from build123d import *

# Parameters (mm, degrees)
F0_W          = 69.85
F0_H          = 6.35
F2_W          = 50.8
F2_H          = 6.35
F5_DEPTH      = 6.35
F7_DEPTH      = 6.35
F9_DEPTH      = 3.8354
F10_T4_DEPTH  = 70.8999806704
F10_T10_DEPTH = 72.2676909626
F11_W         = 69.85
F11_H         = 6.35
F12_DEPTH     = 6.35
F13_W         = 50.8
F13_H         = 6.35
F14_DEPTH     = 50.8
F15_SIZE      = 6.34999
F16_W         = 19.05
F16_H         = 19.05
F17_DEPTH     = 57.15
F18_W         = 19.05
F18_H         = 19.05
F19_DEPTH     = 111.76
F20_SIZE      = 6.34999
F21_R         = 3.175
F22_DEPTH     = 25.4


# Not quite as in the source:
# - a fillet or chamfer that OpenCascade refuses, or shapes differently, is made with other operations: its cross-section is extruded or revolved along the edge and cut away or added
# - a fillet or chamfer is up to 0.001 mm smaller than in the source, because OpenCascade refuses the exact size


with BuildPart() as f3:
    # F0 (on Front) → F3 section 0
    with BuildSketch(Plane.XZ):
        with Locations((-34.925, 3.175)):
            Rectangle(F0_W, F0_H)
    # F2 (on offset) → F3 section 1
    with BuildSketch(Plane.XZ.offset(82.55)):
        with Locations((-34.925, -28.575)):
            Rectangle(F2_W, F2_H)
    loft()

    # F4 (on face) → F5 (join)
    with BuildSketch(Plane(origin=(-68.9322627737, -7.9537226277, 0), x_dir=(0.114624108, -0.9934089359, 0), z_dir=(-0.9934089359, -0.114624108, 0))):
        Polygon((-8.0064939428, 31.75), (-8.0064939428, 6.35), (-8.0064939428, 0), (75.091208342, -31.75), (75.091208342, -25.4), (75.091208342, 0), align=None)
    extrude(amount=F5_DEPTH)

    # F6 (on face) → F7 (join)
    with BuildSketch(Plane(origin=(0, 0, 0), x_dir=(0.114624108, 0.9934089359, 0), z_dir=(0.9934089359, -0.114624108, 0))):
        Polygon((-83.0977022847, 0), (-83.0977022847, -31.75), (0, 0), (0, 31.75), align=None)
    extrude(amount=F7_DEPTH)

    # F8 (on face) → F9 (join)
    with BuildSketch(Plane(origin=(0, -2.1275773196, 5.5317010309), x_dir=(1, 0, 0), z_dir=(0, -0.3589790793, 0.9333456062))):
        Polygon((-61.6927102922, -73.4657484065), (-61.0088551461, -79.8157484065), (-8.8411448539, -79.8157484065), (-8.1572897078, -73.4657484065), align=None)
    extrude(amount=F9_DEPTH)

    # F10: fillet of radius 3.81 on 2 edges, made by hand


with BuildPart() as f10_tool2:
    # F10_s3 → F10_t4 (new body)
    with BuildSketch(Plane.YZ.offset(-70.3749903352)):
        with BuildLine():
            ThreePointArc((-76.6323734692, -23.096775868), (-76.5579487098, -20.1816780202), (-74.4440370018, -18.1730188162))
            Line((-74.4440370018, -18.1730188162), (-78.0000837614, -19.5407291084))
            Line((-78.0000837614, -19.5407291084), (-76.6323734692, -23.096775868))
        make_face()
    extrude(amount=F10_T4_DEPTH)

    split(bisect_by=Plane(origin=(0, 0, 0), x_dir=(0, 0, 1), z_dir=(-0.9934089359, 0.114624108, 0)), keep=Keep.TOP)

    split(bisect_by=Plane(origin=(-68.9322627737, -7.9537226277, 0), x_dir=(0, 0, 1), z_dir=(0.9934089359, 0.114624108, 0)), keep=Keep.TOP)


with BuildPart() as f3_1:
    add(f3.part)

    # F10_t1: cut F10_tool2
    add(f10_tool2.part, mode=Mode.SUBTRACT)


with BuildPart() as f10_tool8:
    # F10_s9 → F10_t10 (new body)
    with BuildSketch(Plane.YZ.offset(1.2088454813)):
        with BuildLine():
            ThreePointArc((-70.7056288698, -20.8172587144), (-72.7142880738, -18.7033470063), (-75.6293859216, -18.6289222469))
            Line((-75.6293859216, -18.6289222469), (-72.073339162, -17.2612119547))
            Line((-72.073339162, -17.2612119547), (-70.7056288698, -20.8172587144))
        make_face()
    extrude(amount=-F10_T10_DEPTH)

    split(bisect_by=Plane(origin=(0, 0, 0), x_dir=(0, 0, 1), z_dir=(-0.9934089359, 0.114624108, 0)), keep=Keep.TOP)

    split(bisect_by=Plane(origin=(-68.9322627737, -7.9537226277, 0), x_dir=(0, 0, 1), z_dir=(0.9934089359, 0.114624108, 0)), keep=Keep.TOP)


with BuildPart() as f3_2:
    add(f3_1.part)

    # F10_t7: cut F10_tool8
    add(f10_tool8.part, mode=Mode.SUBTRACT)

    # F11 (on face) → F12 (join)
    with BuildSketch(Plane(origin=(0, 0, 0), x_dir=(-1, 0, 0), z_dir=(0, 1, 0))):
        with Locations((34.925, 3.175)):
            Rectangle(F11_W, F11_H)
    extrude(amount=F12_DEPTH)

    # F13 (on face) → F14 (join)
    with BuildSketch(Plane.XY.offset(6.35)):
        with Locations((-34.925, 3.175)):
            Rectangle(F13_W, F13_H)
    extrude(amount=F14_DEPTH)

    # F15 (size 6.35 in the source; OpenCascade refuses exactly that, so slightly less here)
    f15_edges = [f3_2.edges().sort_by_distance(p)[0] for p in [
        (-34.925, 0, 57.15),
    ]]
    chamfer(f15_edges, length=F15_SIZE)

    # F16 (on face) → F17 (join)
    with BuildSketch(Plane(origin=(0, 6.35, 0), x_dir=(-1, 0, 0), z_dir=(0, 1, 0))):
        with Locations((34.925, 15.875)):
            Rectangle(F16_W, F16_H)
    extrude(amount=F17_DEPTH)

    # F18 (on face) → F19 (join)
    with BuildSketch(Plane.YZ.offset(-25.4)):
        with Locations((53.975, 15.875)):
            Rectangle(F18_W, F18_H)
    extrude(amount=F19_DEPTH)

    # F20 (size 6.35 in the source; OpenCascade refuses exactly that, so slightly less here)
    f20_edges = [f3_2.edges().sort_by_distance(p)[0] for p in [
        (-65.0875, -41.275, 15.875),
        (-4.7625, -41.275, 15.875),
    ]]
    chamfer(f20_edges, length=F20_SIZE)

    # F21 (on face) → F22 (cut)
    with BuildSketch(Plane.YZ.offset(86.36)):
        with Locations((53.975, 15.875)):
            Circle(F21_R)
    extrude(amount=-F22_DEPTH, mode=Mode.SUBTRACT)


solid = f3_2.part
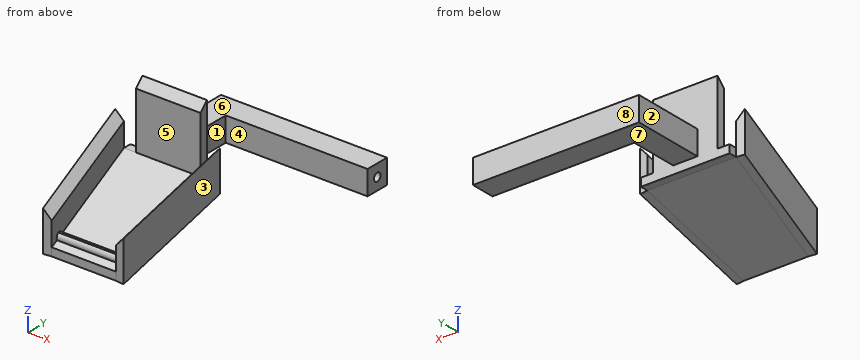
Geometry check sheet. Reference: the model listing, model coordinates, mm. Face numbers are marked on the shaded views. A direction names the side the tool comes from. Round coordinates to 2 decimals unless told otherwise and drop trailing zeros. Write each loop counter-clockwise with the first axis right and the second up, starting at its lowest first coordinate (ties: lowest second). Pieces come first, ordered by that corner, then holes.
Item 1: Section check B-B (x = 23). Record the boundary of the cut face in (y, z).
Determined:
outline: (44.45, 6.35) - (63.5, 6.35) - (63.5, 25.4) - (44.45, 25.4) - close
Item 2: Section check A-A (z = 21.5). Give the number of separate pieces and of enclosed holes in the cut face, plus the area to 3 significant figures.
Determined:
separate pieces: 3
enclosed holes: 0
area: 3,770 mm2
Item 3: Go/stop test with flat-tipped pins: pin 1 Ø7 at (x, y) = (-4.5, 3) entering from +Z; pin 2 Ø8 at (x, y) = (-41, -2.5) entering from +Z; pin 3 Ø5.5 at (y, z) = (21.5, 14) entering from -X. Record where each tip stops, or that it passes through.
Determined:
pin 1: stops at z = 6.35
pin 2: stops at z = 52.3
pin 3: stops at x = -44.45
Item 4: Section check C-C (y = 42.5). Record the boundary of the cut face in (x, z).
Determined:
outline: (-44.45, 6.35) - (-25.4, 6.35) - (-25.4, 25.4) - (-44.45, 25.4) - close
Item 5: Mould release check, pull along Y, two halves, no side actions. Record for the marked faces 1, 2, 3 and 4: +Y half, -Y half, draft (parallel to the pull), parting line (faces both ways), or undercut.
Determined:
face 1: undercut
face 2: draft
face 3: -Y half
face 4: undercut
Item 6: Material ranges on line 1 along X through (y, z) = (48, 10.5); line 2 along Z through (x, y) = (30.5, 51.5); line 3 along X through (y, z) = (-48.5, 0.5), recorded low to high.
Determined:
line 1: x = -44.45 to 86.36
line 2: z = 6.35 to 25.4
line 3: x = -70.65 to -64.25, -5.6 to 0.8
Item 7: Access from +Z, -Z, +X, -X, +Y, -Y to the whole of each face (thin tool, end or side, straight path). Record for the marked faces 5, 6, 7 and 8.
Determined:
face 5: +Z, -Y
face 6: +Z, +X, -X, +Y
face 7: -Z, +X, -X, +Y
face 8: +Z, -Z, +X, -X, +Y
